Geometry check sheet. Reference: drawing and pictorial views, mm from the part's lowest x, y, z. Give positions to 0.01 mm unless a question says otherwise; leave off trailing zeros. Loops run counter-clockwise (first coordinate to the right, second up) from the corner with the lowest first, then second, coordinate; pieces in that order, holes last. Notation, with made-up numbers: (74.25, 55.5) -> (124.25, 55.5) arc R33 cw to (124.25, 94.5) -> close; hole circle Ø1 at (67.5, -33). An arc over 180 degrees is marked (long way). One line per item, written item: value. Start each with the question number.
(1) Scan lines: line 1 along X through (y, z) = (8.5, 3.75); line 2 along Z through (x, y) = (3.5, 9.75) (1 decimal); line 3 along X through (y, z) = (6.25, 4.25). Record each from-to range of solid material in increasing order. Write a range as from..to.
(2) Sectioned sample at D-D, the plane z = 6.25. Record the cut outline in (x, y) (1 decimal).
(3) Sectioned sample at C-C, the plane x = 4.25. Record the cut outline in (y, z) (1 decimal).
(4) Draft check along Z on the marked faces 1, 2 and 3. Enter one of: pulls with the +Z half, pulls with the -Z half, needs draft (parallel to the pull), parting line crosses it, or undercut.
(5) Sectioned sample at B-B, the plane y = 3.25. Record the cut outline in (x, z) (1 decimal).
(6) Sectioned sample at A-A, the plane z = 3. Record the cut outline in (x, y).
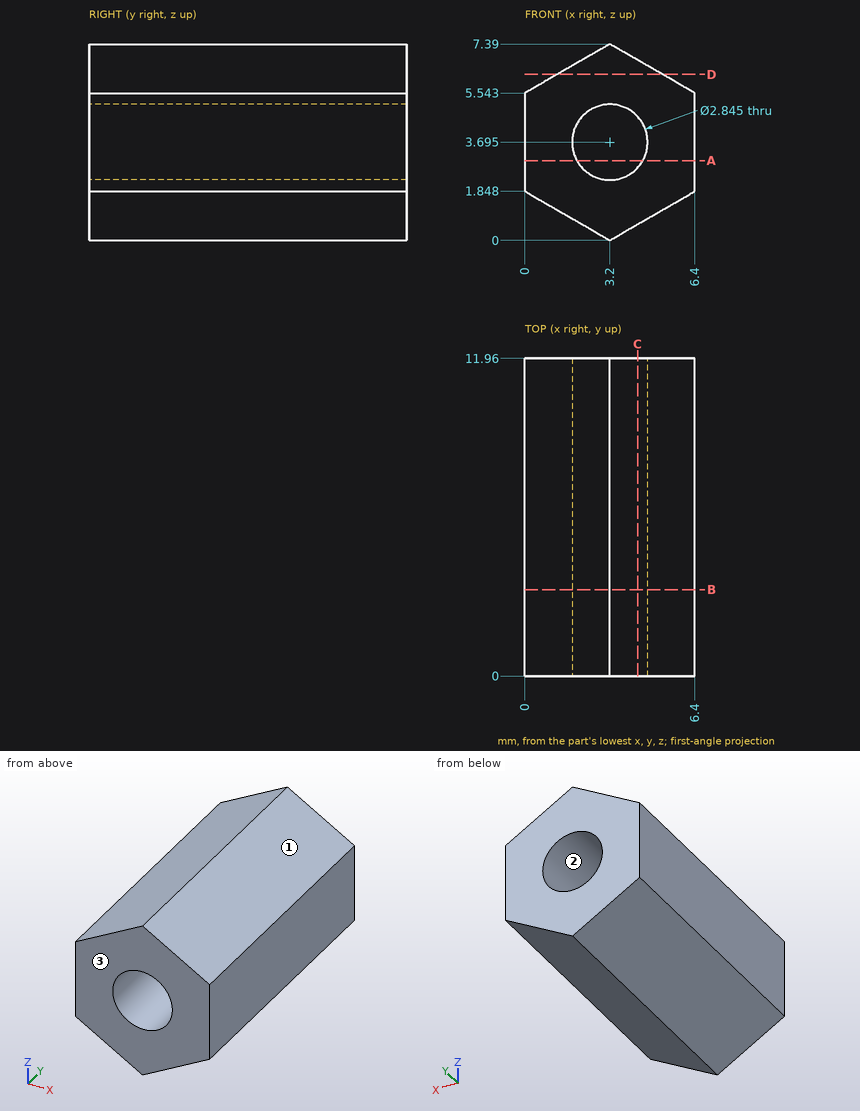
Calculated:
1. line 1: x = 0..1.78, 4.62..6.4
1. line 2: z = 0.2..2.3, 5.1..7.2
1. line 3: x = 0..1.89, 4.51..6.4
2. outline: (1.2, 0) -> (5.2, 0) -> (5.2, 12) -> (1.2, 12) -> close
3. outline: (0, 0.6) -> (12, 0.6) -> (12, 2.7) -> (0, 2.7) -> close; (0, 4.7) -> (12, 4.7) -> (12, 6.8) -> (0, 6.8) -> close
4. face 1: pulls with the +Z half
4. face 2: undercut
4. face 3: needs draft
5. outline: (0, 1.8) -> (3.2, 0) -> (6.4, 1.8) -> (6.4, 5.5) -> (3.2, 7.4) -> (0, 5.5) -> close; hole circle Ø2.8 at (3.2, 3.7)
6. outline: (0, 0) -> (1.96, 0) -> (1.96, 11.96) -> (0, 11.96) -> close; (4.44, 0) -> (6.4, 0) -> (6.4, 11.96) -> (4.44, 11.96) -> close
